```python
from build123d import *
from build123d.topology import SkipClean

# Parameters (mm, degrees)
BOSS_EXTRUDE1_DEPTH = 165.1
SKETCH2_R           = 88.9
BOSS_EXTRUDE2_DEPTH = 63.5
SKETCH3_R           = 127
BOSS_EXTRUDE3_DEPTH = 12.7
BOSS_EXTRUDE4_DEPTH = 209.55
SKETCH6_R           = 76.2
CUT_EXTRUDE1_DEPTH  = 228.6
CUT_EXTRUDE2_REACH  = 433.66
SKETCH7_R           = 19.05
CUT_EXTRUDE3_REACH  = 433.66
SKETCH9_R           = 9.525
CIRPATTERN1_COUNT   = 3


with BuildPart() as part:
    # Sketch1 → Boss-Extrude1 (new body)
    with BuildSketch(Plane.XY):
        with BuildLine():
            Line((-152.4, 0), (152.4, 0))
            Line((152.4, 0), (82.285119295, 171.45))
            ThreePointArc((82.285119295, 171.45), (0, 226.699306951), (-82.285119295, 171.45))
            Line((-82.285119295, 171.45), (-152.4, 0))
        make_face()
    extrude(amount=BOSS_EXTRUDE1_DEPTH)

    # Sketch2 → Boss-Extrude2 (add)
    with BuildSketch(Plane.XY.offset(165.1)):
        with Locations(Location((0, 137.799306951, 0), (0, 0, 157.757777303))):
            Circle(SKETCH2_R)
    extrude(amount=BOSS_EXTRUDE2_DEPTH)

    # Sketch3 → Boss-Extrude3 (add)
    with BuildSketch(Plane.XY.offset(228.6)):
        with Locations((0, 137.799306951)):
            Circle(SKETCH3_R)
    extrude(amount=BOSS_EXTRUDE3_DEPTH)

    # Sketch4 → Boss-Extrude4 (add)
    with SkipClean():  # the faces are left unmerged after this step: merging them gives an invalid solid
        with BuildSketch(Plane(origin=(0, 0, 19.05), x_dir=(-1, 0, 0), z_dir=(0, 0, -1))):
            with BuildLine():
                Line((-63.5, 189.570098967), (-63.5, 243.84))
                Line((-63.5, 243.84), (-76.2, 243.84))
                Line((-76.2, 243.84), (-76.2, 255.27))
                Line((-76.2, 255.27), (-63.5, 255.27))
                Line((-63.5, 255.27), (-63.5, 266.7))
                Line((-63.5, 266.7), (-76.2, 266.7))
                Line((-76.2, 266.7), (-76.2, 278.13))
                Line((-76.2, 278.13), (-63.5, 278.13))
                Line((-63.5, 278.13), (-63.5, 289.56))
                Line((-63.5, 289.56), (-76.2, 289.56))
                Line((-76.2, 289.56), (-76.2, 300.99))
                Line((-76.2, 300.99), (-63.5, 300.99))
                Line((-63.5, 300.99), (-63.5, 312.42))
                Line((-63.5, 312.42), (-76.2, 312.42))
                Line((-76.2, 312.42), (-76.2, 323.85))
                Line((-76.2, 323.85), (76.2, 323.85))
                Line((76.2, 323.85), (76.2, 312.42))
                Line((76.2, 312.42), (63.5, 312.42))
                Line((63.5, 312.42), (63.5, 300.99))
                Line((63.5, 300.99), (76.2, 300.99))
                Line((76.2, 300.99), (76.2, 289.56))
                Line((76.2, 289.56), (63.5, 289.56))
                Line((63.5, 289.56), (63.5, 278.13))
                Line((63.5, 278.13), (76.2, 278.13))
                Line((76.2, 278.13), (76.2, 266.7))
                Line((76.2, 266.7), (63.5, 266.7))
                Line((63.5, 266.7), (63.5, 255.27))
                Line((63.5, 255.27), (76.2, 255.27))
                Line((76.2, 255.27), (76.2, 243.84))
                Line((76.2, 243.84), (63.5, 243.84))
                Line((63.5, 243.84), (63.5, 189.570098967))
                ThreePointArc((63.5, 189.570098967), (0, 219.728940821), (-63.5, 189.570098967))
            make_face()
        extrude(amount=-BOSS_EXTRUDE4_DEPTH)

    # Sketch6 → Cut-Extrude1 (cut)
    with SkipClean():  # the faces are left unmerged after this step: merging them gives an invalid solid
        with BuildSketch(Plane.XY.offset(241.3)):
            with Locations((0, 137.799306951)):
                Circle(SKETCH6_R)
        extrude(amount=-CUT_EXTRUDE1_DEPTH, mode=Mode.SUBTRACT)

    # Sketch7 → Cut-Extrude2 (cut, up to next)
    with BuildSketch(Plane(origin=(0, 0, 0), x_dir=(-1, 0, 0), z_dir=(0, 0, -1)), mode=Mode.PRIVATE) as cut_extrude2_sk1:
        with Locations((0, 137.799306951)):
            Circle(SKETCH7_R)
    cut_extrude2_tool1 = extrude(cut_extrude2_sk1.sketch, amount=-CUT_EXTRUDE2_REACH, mode=Mode.PRIVATE) & part.part
    add(cut_extrude2_tool1.solids().sort_by_distance((0, 137.799307, 0))[0], mode=Mode.SUBTRACT)

    # Sketch9 → Cut-Extrude3 (cut, up to next)
    with BuildSketch(Plane.XY.offset(241.3), mode=Mode.PRIVATE) as cut_extrude3_sk1:
        with Locations((0, 29.849306951)):
            Circle(SKETCH9_R)
    cut_extrude3_tool1 = extrude(cut_extrude3_sk1.sketch, amount=-CUT_EXTRUDE3_REACH, mode=Mode.PRIVATE) & part.part
    cut_extrude3 = cut_extrude3_tool1.solids().sort_by_distance((0, 29.849307, 241.3))[0]
    add(cut_extrude3, mode=Mode.SUBTRACT)

    # CirPattern1: Cut-Extrude3 ×3 about axis
    with SkipClean():  # the faces are left unmerged after this step: merging them gives an invalid solid
        cirpattern1_axis = Axis((0, 137.799306951, 0), (0, 0, 1))
        for i in range(1, CIRPATTERN1_COUNT):
            add(cut_extrude3.rotate(cirpattern1_axis, i * 360 / CIRPATTERN1_COUNT), mode=Mode.SUBTRACT)


solid = part.part
```
Geometry: final body of the model. Coordinates: model frame, mm. A direction names the side the tool comes from. Round coordinates to 2 decimals unless told otherwise and drop trailing zeros. Write each loop counter-clockwise with the first axis right and the second up, starting at its lowest first coordinate (ties: lowest second). Pieces come first, ordered by that corner, then holes. Notation, with made-up numbers: M 10.5,-26.75 L 50.5,-26.75 A17 cw 50.5,-22.75 Z; hole C 89,1.25 d2. An arc over 180 degrees is marked long. Answer in a Markdown table with one row per item. Add a question column.
(1) Cut plane C-C, the plane x = -112. Return the cut outline in (y, z), then the cut area to 3 significant figures.
(2) Reachability of faces 4 (the face through (-63.5, 222, 122)), 5 (the face through (70, 255.27, 122)), 6 (the face through (76.2, 272, 122)), 7 (the face through (-70, 255.27, 122)), 8 (the face through (-2.06, 20.55, 235.04)) from +Z, -Z, +X, -X, +Y, -Y: full face, straight path, thin tool, end or side. Return the list, or none.
(3) Contact query for flat-ended pins moving along their axis: pin 1 (9 mm diameter, centred on y = 297, z = 164, fed in from +X); pin 2 (9 mm diameter, centred on y = 298, z = 151, fed in from -X); pin 3 (2 mm diameter, centred on y = 34, z = 72.5, fed in from -X). Output: stop coordinate, or through.
(4) Draft query along Y for faces 1 (the face through (1, 323.85, 122)), 2 (the face through (76.2, 249, 122)), 3 (the face through (63.5, 261, 122)). Return one class per face: pulls with the +Y half, pulls with the -Y half, needs draft (parallel to the pull), parting line crosses it, or undercut.
(5) Ray query, L1, parallel to Y at x = 0, z = 238.75; L2, parallel to Z at x = -83, y = 47; L3, parallel to Y at x = 0, z = 91. Return the intervals inside material, ascending.
(6) Cut plane A-A, the plane x = 0. Return the cut outline in (y, z).
Established:
| question | item | result |
|---|---|---|
| 1 | outline | M 0,0 L 98.79,0 L 98.79,165.1 L 0,165.1 Z; M 77.92,228.6 L 197.67,228.6 L 197.67,241.3 L 77.92,241.3 Z |
| 1 | area | 17,800 mm² |
| 2 | face 4 | -Z, -X |
| 2 | face 5 | +Z, -Z, +X |
| 2 | face 6 | +Z, -Z, +X, +Y |
| 2 | face 7 | +Z, -Z, -X |
| 2 | face 8 | +Z |
| 3 | pin 1 | x = 76.2 |
| 3 | pin 2 | x = -76.2 |
| 3 | pin 3 | x = -138.9 |
| 4 | face 1 | pulls with the +Y half |
| 4 | face 2 | needs draft |
| 4 | face 3 | undercut |
| 5 | L1 | 10.8 to 20.32, 39.37 to 61.6, 214 to 264.8 |
| 5 | L2 | 0 to 165.1, 228.6 to 241.3 |
| 5 | L3 | 0 to 61.6, 214 to 323.85 |
| 6 | outline | M 0,0 L 118.75,0 L 118.75,12.7 L 61.6,12.7 L 61.6,241.3 L 39.37,241.3 L 39.37,228.6 L 48.9,228.6 L 48.9,165.1 L 0,165.1 Z; M 10.8,228.6 L 20.32,228.6 L 20.32,241.3 L 10.8,241.3 Z; M 156.85,0 L 226.7,0 L 226.7,19.05 L 323.85,19.05 L 323.85,228.6 L 264.8,228.6 L 264.8,241.3 L 214,241.3 L 214,12.7 L 156.85,12.7 Z |
